```python
from build123d import *

# Parameters (mm, degrees)
BOSS_EXTRUDE2_DEPTH = 88.9
SKETCH19_R          = 2.032
CUT_EXTRUDE3_DEPTH  = 94.922403297


with BuildPart() as part:
    # Sketch2 → Boss-Extrude2 (new body)
    with BuildSketch(Plane.XY):
        Polygon((0, 0), (0, 20.32), (22.479, 20.32), (22.479, 0), (19.304, 0), (19.304, 16.129), (3.175, 16.129), (3.175, 0), align=None)
    extrude(amount=-BOSS_EXTRUDE2_DEPTH)

    # Sketch19 → Cut-Extrude3 (cut, through all)
    with BuildSketch(Plane(origin=(0, 0, 0), x_dir=(0, 0, -1), z_dir=(1, 0, 0))):
        with Locations((24.13, 14.224)):
            Circle(SKETCH19_R)
        with Locations((64.77, 14.224)):
            Circle(SKETCH19_R)
    extrude(amount=CUT_EXTRUDE3_DEPTH, mode=Mode.SUBTRACT)


solid = part.part
```
Could you check a few things on this model? Use its own coordinates, in mm. A direction names the side the tool comes from. Coordinates: 2 decimals unless noted, no trailing zeros. Write each loop counter-clockwise with the first axis right and the second up, starting at its lowest first coordinate (ties: lowest second). Pieces come first, ordered by that corner, then holes. Notation, with made-up numbers: (71, 48) -> (97, 48) arc R31 cw to (97, 72) -> close; hole circle Ø10 at (0, 3.25). An arc over 180 degrees is marked (long way). Write item = value, one per line. Start each with the question number.
(1) Will this pin go through, and if not, where does the flat tip stop? pin 1 (8 mm diameter, centred on x = 15, z = -38, fed in from -Y).
(2) Which directions (+Z, -Z, +X, -X, +Y, -Y) give clear straight access to the entire face, cutting with the end or side of a thin tool? Please do faces 1 (the face through (2, 0, -44)), 2 (the face through (11, 16.129, -77)).
(3) I want a section at A-A (y = 4.25). Please give me the cut outline in (x, z) (3 decimals), plus the area to 3 significant figures.
(4) I want a section at C-C (x = 13.5). Please give me the cut outline in (y, z), plus the area to 3 significant figures.
(5) I need wall thicknesses on line 1 (X direction, y = 11.75, z = -33) (3 decimals); line 2 (Z direction, x = 19.75, y = 15.5); line 3 (Y direction, x = 7.25, z = -64.77). Which ranges of each line are inside material? Lowest first, please. Write a range as [from, to].
(6) I want a section at B-B (z = -33.5). Please give me the cut outline in (x, y) (3 decimals).
(7) We'd pull the mould along Z, two halves only. Please class faces 3 (the face through (11, 17, 0)), 4 (the face through (11, 17, -88.9)), 5 (the face through (22.479, 10, -44)), 6 (the face through (12.02, 16.25, -24.28)): released by +Z, released by -Z, zero draft, split by the parting line, or undercut.
Result set:
q1.pin_1 = 16.13
q2.face_1 = +Z, -Z, +X, -X, -Y
q2.face_2 = +Z, -Z, -Y
q3.outline = (0, -88.9) -> (3.175, -88.9) -> (3.175, 0) -> (0, 0) -> close; (19.304, -88.9) -> (22.479, -88.9) -> (22.479, 0) -> (19.304, 0) -> close
q3.area = 565 mm2
q4.outline = (16.13, -88.9) -> (20.32, -88.9) -> (20.32, 0) -> (16.13, 0) -> (16.13, -23.42) arc R2.03 cw to (16.13, -24.84) -> (16.13, -64.06) arc R2.03 cw to (16.13, -65.48) -> close
q4.area = 372 mm2
q5.line_1 = [0, 3.175], [19.304, 22.479]
q5.line_2 = [-88.9, -66.35], [-63.19, -25.71], [-22.55, 0]
q5.line_3 = [16.26, 20.32]
q6.outline = (0, 0) -> (3.175, 0) -> (3.175, 16.129) -> (19.304, 16.129) -> (19.304, 0) -> (22.479, 0) -> (22.479, 20.32) -> (0, 20.32) -> close
q7.face_3 = released by +Z
q7.face_4 = released by -Z
q7.face_5 = zero draft
q7.face_6 = undercut
